Verification items for this drawing (mm, ordinates from the low corner). A direction names the side the tool comes from. Round coordinates to 2 decimals unless told otherwise and drop trailing zeros. Write each loop counter-clockwise with the first axis right and the second up, starting at its lowest first coordinate (ties: lowest second). Pieces come first, ordered by that corner, then holes. Notation, with made-up numbers: M 85.25,23 L 93.25,23 A13 cw 93.25,41 Z; hole C 16,21 d4. An arc over 180 degrees is marked long. One line per question, with ' | ' between items. Start each with the question number.
Q1. Cross-section at A-A (z = 10.75). Record the boundary of the cut face in (x, y), then the cut area to 3 significant figures.
Q2. Thickness scan on line 1 along X through (y, z) = (4.05, 19.4); line 2 along Y through (x, z) = (21.5, 19.75); line 3 along X through (y, z) = (2, 1.75). Record the ranges inside material, lowest first. Write a range as from..to.
Q3. Tool access check on the marked faces 5 and 6. Record the directions out of +Z, -Z, +X, -X, +Y, -Y that give a thin tool (end or side, any length) a straight path to the whole face; none if there is none.
Q4. Cross-section at D-D (y = 1.25). Record the boundary of the cut face in (x, z).
Q5. Gauge pin test, flat ends, axial feed: pin 1 (12 mm diameter, centred on x = 22, z = 12, fed in from +Y); pin 2 (8 mm diameter, centred on x = 17, z = 10.5, fed in from +Y); pin 3 (4 mm diameter, centred on x = 12.5, y = 1.5, fed in from -Z). Record the tip position at first contact, or that the pin passes through.
Q6. Cross-section at B-B (y = 4.05). Record the boundary of the cut face in (x, z).
Q7. Release check for a two-part mould opening along X. For the marked faces 1, 2, 3 and 4 record: released by +X, released by -X, zero draft, split by the parting line, or undercut.
Q8. Cross-section at C-C (x = 21.5). Record the boundary of the cut face in (y, z), then the cut area to 3 significant figures.
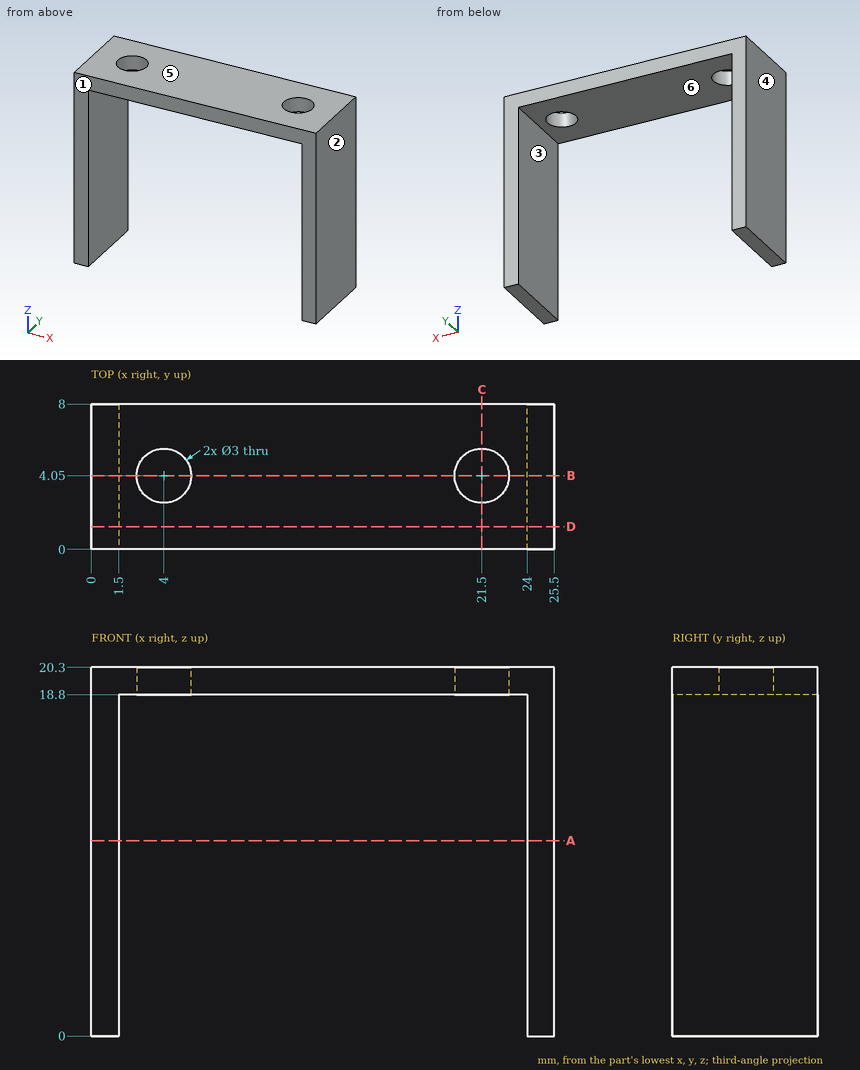
Determined:
1) outline: M 0,0 L 1.5,0 L 1.5,8 L 0,8 Z; M 24,0 L 25.5,0 L 25.5,8 L 24,8 Z | area: 24.0 mm²
2) line 1: x = 0..2.5, 5.5..20, 23..25.5 | line 2: y = 0..2.55, 5.55..8 | line 3: x = 0..1.5, 24..25.5
3) face 5: +Z, +X, -X, +Y, -Y | face 6: -Z, +Y, -Y
4) outline: M 0,0 L 1.5,0 L 1.5,18.8 L 24,18.8 L 24,0 L 25.5,0 L 25.5,20.3 L 0,20.3 Z
5) pin 1: stops at y = 8 | pin 2: passes through | pin 3: stops at z = 18.8
6) outline: M 0,0 L 1.5,0 L 1.5,18.8 L 2.5,18.8 L 2.5,20.3 L 0,20.3 Z; M 5.5,18.8 L 20,18.8 L 20,20.3 L 5.5,20.3 Z; M 23,18.8 L 24,18.8 L 24,0 L 25.5,0 L 25.5,20.3 L 23,20.3 Z
7) face 1: zero draft | face 2: released by +X | face 3: undercut | face 4: released by -X
8) outline: M 0,18.8 L 2.55,18.8 L 2.55,20.3 L 0,20.3 Z; M 5.55,18.8 L 8,18.8 L 8,20.3 L 5.55,20.3 Z | area: 7.50 mm²
